from build123d import *

# Parameters (mm, degrees)
SKETCH1_R           = 2.5
BOSS_EXTRUDE1_DEPTH = 3


with BuildPart() as part:
    # Sketch1 → Boss-Extrude1 (new body)
    with BuildSketch(Plane.XY):
        Polygon((60.2, 197), (60.2, 200), (40, 200), (40, 197), (20.2, 197), (20.2, 200), (0, 200), (0, 169.9), (3, 169.9), (3, 150.1), (0, 150.1), (0, 129.9), (3, 129.9), (3, 110.1), (0, 110.1), (0, 89.9), (3, 89.9), (3, 70.1), (0, 70.1), (0, 49.9), (3, 49.9), (3, 30.1), (0, 30.1), (0, 0), (20.2, 0), (20.2, 3), (40, 3), (40, 0), (60.2, 0), (60.2, 3), (80, 3), (80, 0), (100, 0), (100, 30.1), (97, 30.1), (97, 49.9), (100, 49.9), (100, 70.1), (97, 70.1), (97, 89.9), (100, 89.9), (100, 110.1), (97, 110.1), (97, 129.9), (100, 129.9), (100, 150.1), (97, 150.1), (97, 169.9), (100, 169.9), (100, 200), (80, 200), (80, 197), align=None)
        with Locations((50, 100)):
            Circle(SKETCH1_R, mode=Mode.SUBTRACT)
    extrude(amount=BOSS_EXTRUDE1_DEPTH)


solid = part.part
Geometry: final body of the model. Coordinates: model frame, mm. Round coordinates to 2 decimals unless told otherwise and drop trailing zeros. Loops run counter-clockwise (first coordinate to the right, second up) from the corner with the lowest first, then second, coordinate; pieces in that order, holes last. Notation, with made-up numbers: M -36.75,17 L -29.75,17 A24 cw -29.75,36 Z; hole C -26,63 d10. An arc over 180 degrees is marked long. Put each result on its own line as item: value. Start each with the question number.
(1) Material intervals for line 1 along Y through (x, z) = (50, 0.7); line 2 along Y through (x, z) = (69.5, 2.5); line 3 along X through (y, z) = (127, 0.95), sorted ascending. Write a range as [from, to].
(2) Section query B-B (y = 100). Return loops of the section in (x, z).
(3) Draft query along X for faces 1 (the face through (38, 101, 0)), 2 (the face through (49.67, 102.48, 1.48)). Return one class per face: +X half, -X half, draft (parallel to the pull), parting line (faces both ways), or undercut.
(4) Contact query for flat-ended pins moving along their axis: pin 1 Ø0.9 at (y, z) = (116, 1.5) entering from -X; pin 2 Ø1.5 at (y, z) = (40, 1) entering from +X. Output: stop coordinate, or through.
(5) Section query C-C (x = 29). Return loops of the section in (y, z), then the cut area to 3 significant figures.
(6) Section query A-A (x = 50). Return loops of the section in (y, z).
Findings below:
1. line 1: y = [0, 97.5], [102.5, 200]
1. line 2: y = [3, 197]
1. line 3: x = [3, 97]
2. outline: M 0,0 L 47.5,0 L 47.5,3 L 0,3 Z; M 52.5,0 L 100,0 L 100,3 L 52.5,3 Z
3. face 1: draft
3. face 2: undercut
4. pin 1: stops at x = 3
4. pin 2: stops at x = 97
5. outline: M 3,0 L 197,0 L 197,3 L 3,3 Z
5. area: 582 mm2
6. outline: M 0,0 L 97.5,0 L 97.5,3 L 0,3 Z; M 102.5,0 L 200,0 L 200,3 L 102.5,3 Z
